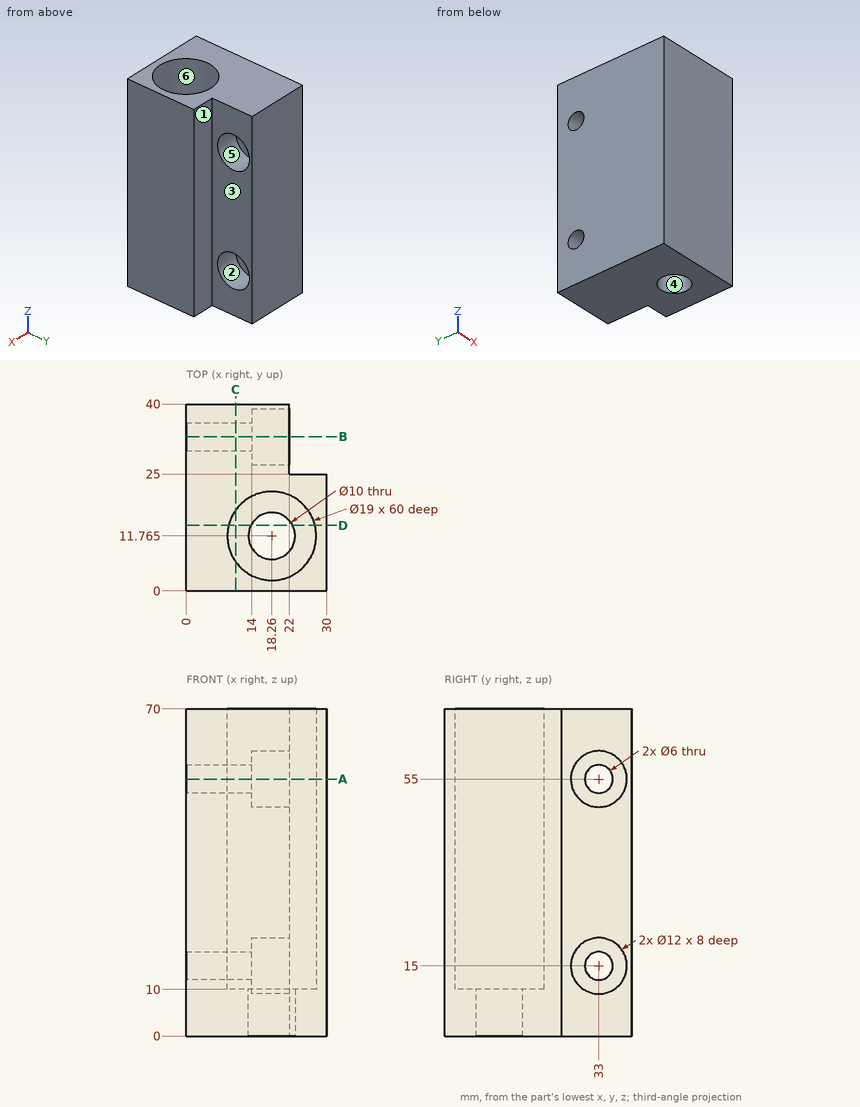
Geometry check sheet. Reference: drawing and pictorial views, mm from the part's lowest x, y, z. A direction names the side the tool comes from. Coordinates: 2 decimals unless noted, no trailing zeros. Loops run counter-clockwise (first coordinate to the right, second up) from the corner with the lowest first, then second, coordinate; pieces in that order, holes last. Notation, with made-up numbers: (45, -29.5) -> (62, -29.5) arc R28 cw to (62, 5.5) -> close; hole circle Ø7 at (7, -28.5). An arc over 180 degrees is marked (long way). Put each result on its own line as item: value.
1) Cross-section at D-D on y = 14. Record the boundary of the cut face in (x, z).
Result set:
outline: (0, 0) -> (13.79, 0) -> (13.79, 10) -> (9.03, 10) -> (9.03, 70) -> (0, 70) -> close; (22.73, 0) -> (30, 0) -> (30, 70) -> (27.49, 70) -> (27.49, 10) -> (22.73, 10) -> close
2) Tool access check on the marked faces 4, 5 and 6. Record the directions out of +Z, -Z, +X, -X, +Y, -Y that give a thin tool (end or side, any length) a straight path to the whole face; none if there is none.
Result set:
face 4: +Z, -Z
face 5: +X
face 6: +Z
3) Cross-section at C-C on x = 10.5. Record the boundary of the cut face in (y, z) (1 decimal).
Result set:
outline: (0, 0) -> (40, 0) -> (40, 70) -> (17.2, 70) -> (17.2, 10) -> (6.3, 10) -> (6.3, 70) -> (0, 70) -> close; hole circle Ø6 at (33, 15); hole circle Ø6 at (33, 55)
4) Cross-section at B-B on y = 33. Record the boundary of the cut face in (x, z).
Result set:
outline: (0, 0) -> (22, 0) -> (22, 9) -> (14, 9) -> (14, 12) -> (0, 12) -> close; (0, 18) -> (14, 18) -> (14, 21) -> (22, 21) -> (22, 49) -> (14, 49) -> (14, 52) -> (0, 52) -> close; (0, 58) -> (14, 58) -> (14, 61) -> (22, 61) -> (22, 70) -> (0, 70) -> close
5) Thickness scan on line 1 (Y direction, x = 17, z = 15); line 2 (Z direction, x = 21.5, y = 35.5) (1 decimal); line 3 (Y direction, x = 18, z = 15). Record the ranges inside material, lowest first.
Result set:
line 1: y = 0 to 2.35, 21.18 to 27, 39 to 40
line 2: z = 0 to 9.5, 20.5 to 49.5, 60.5 to 70
line 3: y = 0 to 2.27, 21.26 to 27, 39 to 40
6) Cross-section at A-A on z = 55. Record the boundary of the cut face in (x, y) (1 decimal).
Result set:
outline: (0, 0) -> (30, 0) -> (30, 25) -> (22, 25) -> (22, 27) -> (14, 27) -> (14, 30) -> (0, 30) -> close; (0, 36) -> (14, 36) -> (14, 39) -> (22, 39) -> (22, 40) -> (0, 40) -> close; hole circle Ø19 at (18.3, 11.8)
7) Release check for a two-part mould opening along Y. For the marked faces 1, 2 and 3 record: released by +Y, released by -Y, zero draft, split by the parting line, or undercut.
Result set:
face 1: released by +Y
face 2: undercut
face 3: zero draft
8) Gauge pin test, flat ends, axial feed: pin 1 Ø1.5 at (y, z) = (35.5, 57.5) entering from +X; pin 2 Ø13 at (x, y) = (18.26, 11.77) entering from +Z; pin 3 Ø2.5 at (x, z) = (27.5, 21.5) entering from +Y; pin 4 Ø3.5 at (y, z) = (33, 15) entering from -X. Record the tip position at first contact, or that the pin passes through.
Result set:
pin 1: stops at x = 14
pin 2: stops at z = 10
pin 3: stops at y = 25
pin 4: passes through
